For this review, take the finished solid that the model builds, in its own axes (mm). A direction names the side the tool comes from. Give positions to 0.01 mm unless a question says otherwise; leave off trailing zeros. Write each loop counter-clockwise with the first axis right and the second up, starting at its lowest first coordinate (ties: lowest second). Pieces come first, ordered by that corner, then holes. Notation, with made-up numbers: M -30.75,-39.5 L -26.75,-39.5 A22 cw -26.75,-33.5 Z; hole C -5,-15.75 d10. An arc over 180 degrees is marked long. Answer as a JSON object with one key per item and string values. Group by question number.
```python
from build123d import *

# Parameters (mm, degrees)
SKETCH1_W             = 130
SKETCH1_H             = 100
BOSS_EXTRUDE1_DEPTH   = 15
SKETCH2_R             = 45.5
BOSS_EXTRUDE2_DEPTH   = 90
SKETCH3_R             = 41
CUT_EXTRUDE1_DEPTH    = 106
SKETCH4_R             = 42.5
CUT_EXTRUDE2_DEPTH    = 55
M8_TAPPED_HOLE1_D     = 6.8
M8_TAPPED_HOLE1_DEPTH = 17.707073895
M8_TAPPED_HOLE1_TIP   = 2.042926105
SKETCH11_R            = 2.5
CUT_EXTRUDE3_DEPTH    = 106


with BuildPart() as part:
    # Sketch1 → Boss-Extrude1 (new body)
    with BuildSketch(Plane(origin=(0, 0, 0), x_dir=(1, 0, 0), z_dir=(0, 1, 0))):
        Rectangle(SKETCH1_W, SKETCH1_H)
    extrude(amount=BOSS_EXTRUDE1_DEPTH)

    # Sketch2 → Boss-Extrude2 (add)
    with BuildSketch(Plane(origin=(0, 15, 0), x_dir=(1, 0, 0), z_dir=(0, 1, 0))):
        Circle(SKETCH2_R)
    extrude(amount=BOSS_EXTRUDE2_DEPTH)

    # Sketch3 → Cut-Extrude1 (cut, through all)
    with BuildSketch(Plane(origin=(0, 105, 0), x_dir=(1, 0, 0), z_dir=(0, 1, 0))):
        Circle(SKETCH3_R)
    extrude(amount=-CUT_EXTRUDE1_DEPTH, mode=Mode.SUBTRACT)

    # Sketch4 → Cut-Extrude2 (cut)
    with BuildSketch(Plane.XZ):
        Circle(SKETCH4_R)
    extrude(amount=-CUT_EXTRUDE2_DEPTH, mode=Mode.SUBTRACT)

    # M8 Tapped Hole1
    with Locations(Plane(origin=(0, 15, 0), x_dir=(1, 0, 0), z_dir=(0, 1, 0))):
        with Locations((-50, 23.25), (-50, -23.25), (50, -23.25), (50, 23.25)):
            Hole(M8_TAPPED_HOLE1_D / 2, depth=M8_TAPPED_HOLE1_DEPTH)
            with Locations((0, 0, -(M8_TAPPED_HOLE1_DEPTH + M8_TAPPED_HOLE1_TIP / 2))):  # 118° drill point
                Cone(0, M8_TAPPED_HOLE1_D / 2, M8_TAPPED_HOLE1_TIP, mode=Mode.SUBTRACT)

    # Sketch11 → Cut-Extrude3 (cut, through all)
    with BuildSketch(Plane.XZ):
        with Locations((-59, 14.25)):
            Circle(SKETCH11_R)
        with Locations((59, -14.25)):
            Circle(SKETCH11_R)
    extrude(amount=-CUT_EXTRUDE3_DEPTH, mode=Mode.SUBTRACT)


solid = part.part
```
Item 1: Consider section C-C (x = 4.5). Give the boundary of the cut face in (y, z), plus the area to 3 significant figures.
Item 2: Draft analysis for pull direction X (two halves, no side actions). For faces 1 (the cylindrical face through (-53.14, 7.4, -21.95)), 2 (the flat face through (-65, 7, 1)), 3 (the flat face through (-44.2, 15, -11.8)), state which applies: released by +X, released by -X, zero draft, split by the parting line, or undercut.
Item 3: Consider section D-D (z = -23.25). Give the boundary of the cut face in (x, y), plus the area to 3 significant figures.
Item 4: Consider section B-B (z = 31). Give the boundary of the cut face in (x, y), plus the area to 3 significant figures.
Item 5: Machinability: for faces 4 (the cylindrical face through (-36.107, 59.37, 27.686)), 5 (the flat face through (-22, 55, 35)), 6 (the flat face through (-44, 0, -1)), which of the approach directions +Z, -Z, +X, -X, +Y, -Y give a long, thin tool a straight path to every point of the face, cutting with its end or side? Answer none if there is none.
Item 6: To check wall thickness, follow probe 1 along Z at (x, y) = (-50, 10); probe 2 along Z at (x, y) = (-59, 9.5); probe 3 along X at (y, z) = (4, 23.25). State the ranges of each line that lie inside material, in increasing order.
Item 7: Consider section A-A (x = 50). Give the boundary of the cut face in (y, z).
Item 8: Insertion check: P1, Ø1.5, axis at x = -31.5, y = 73.5, coming from the +Z side; P2, Ø11, axis at x = 50, z = 23.25, coming from the +Y side; P3, Ø6, axis at x = 41, y = 55.5, coming from the +Z side (3 decimals). Each pin has a flat end and moves straight along its axis. Give the tip position at first contact, or say it passes through.
Result set:
{
 "1": {"outline": "M 0,-50 L 15,-50 L 15,-45.28 L 105,-45.28 L 105,-40.75 L 55,-40.75 L 55,-42.26 L 0,-42.26 Z; M 0,42.26 L 55,42.26 L 55,40.75 L 105,40.75 L 105,45.28 L 15,45.28 L 15,50 L 0,50 Z", "area": "926 mm^2"},
 "2": {"face 1": "undercut", "face 2": "released by -X", "face 3": "zero draft"},
 "3": {"outline": "M -65,0 L -53.4,0 L -53.4,15 L -65,15 Z; M -46.6,0 L -35.58,0 L -35.58,55 L -33.77,55 L -33.77,105 L -39.11,105 L -39.11,15 L -46.6,15 Z; M 33.77,55 L 35.58,55 L 35.58,0 L 46.6,0 L 46.6,15 L 39.11,15 L 39.11,105 L 33.77,105 Z; M 53.4,0 L 65,0 L 65,15 L 53.4,15 Z", "area": "1,500 mm^2"},
 "4": {"outline": "M -65,0 L -29.07,0 L -29.07,55 L -26.83,55 L -26.83,105 L -33.31,105 L -33.31,15 L -65,15 Z; M 26.83,55 L 29.07,55 L 29.07,0 L 65,0 L 65,15 L 33.31,15 L 33.31,105 L 26.83,105 Z", "area": "2,060 mm^2"},
 "5": {"face 4": "+Y", "face 5": "-Y", "face 6": "+Z, -Z, +X, -X, -Y"},
 "6": {"probe 1": "z = -50 to -26.65, -19.85 to 19.85, 26.65 to 50", "probe 2": "z = -50 to 11.75, 16.75 to 50", "probe 3": "x = -65 to -53.4, -46.6 to -35.58, 35.58 to 46.6, 53.4 to 65"},
 "7": {"outline": "M 0,-50 L 15,-50 L 15,-26.65 L 0,-26.65 Z; M 0,-19.85 L 15,-19.85 L 15,19.85 L 0,19.85 Z; M 0,26.65 L 15,26.65 L 15,50 L 0,50 Z"},
 "8": {"P1": "stops at z = 33.54", "P2": "stops at y = 15", "P3": "stops at z = 25.025"}
}
